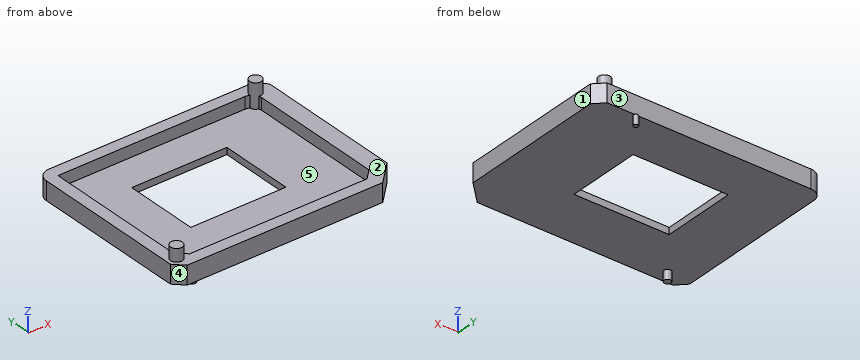
Autodesk Inventor part; units mm, degrees
ref_plane "YZ Plane" through (0, 0, 0) normal (1, 0, 0) x (0, 1, 0)
ref_plane "XZ Plane" through (0, 0, 0) normal (0, 1, 0) x (-1, 0, 0)
ref_plane "XY Plane" through (0, 0, 0) normal (0, 0, 1) x (1, 0, 0)
sketch "Sketch1" plane through (0, 0, 0) normal (0, 0, 1) x (1, 0, 0)
  line L0 (2, 0) -> (43.86, 0)
  line L1 (48.26, 4.4) -> (48.26, 36.1)
  line L2 (46.26, 38.1) -> (2.6, 38.1)
  line L3 (0, 35.5) -> (0, 2)
  arc A0 (2.6, 38.1) -> (0, 35.5) centre (2.6, 35.5) ccw
  line L4 (2.54, 35.56) -> (42.54, 35.56)
  line L5 (44.54, 33.56) -> (44.54, 4.56)
  line L6 (42.54, 2.56) -> (4.54, 2.56)
  line L7 (2.54, 4.56) -> (2.54, 35.56)
  line L8 (43.86, 0) -> (48.26, 4.4)
  line L9 (44.54, 4.56) -> (42.54, 2.56)
  line L10 (4.54, 2.56) -> (2.54, 4.56)
  circle A1 centre (44.72, 35.43) radius 1.28
  circle A2 centre (1.97, 2.85) radius 1.27
  line L11 (2.54, 35.56) -> (44.54, 2.56) construction
  line L12 (44.54, 35.56) -> (2.54, 2.56) construction
  arc A3 (44.54, 33.56) -> (42.54, 35.56) centre (42.54, 33.56) ccw
  line L13 (48.26, 36.1) -> (46.26, 38.1)
  line L14 (2, 0) -> (0, 2)
  point P0 (0, 0)
  point P1 (48.26, 38.1)
  point P2 (48.26, 0)
  point P3 (0, 38.1)
  point P4 (4.2502, 2.8498)
  point P5 (2.916, 4.184)
  point P6 (43.4429, 35.3446)
  point P7 (44.4412, 34.1807)
  dimension "d0" = 38.1
  dimension "d1" = 48.26
  dimension "d2" = 2.6
  dimension "d3" = 33
  dimension "d4" = 42
  dimension "d5" = 2.54
  dimension "d6" = 2.54
  dimension "d7" = 4.4
  dimension "d8" = 4.4
  dimension "d9" = 2
  dimension "d10" = 2
  dimension "d11" = 2
  dimension "d12" = 2
  dimension "d13" = 44.72
  dimension "d14" = 2.56
  dimension "d15" = 2.67
  dimension "d16" = 2.54
  dimension "d27" = 2
  dimension "d28" = 2
  dimension "d29" = 2
  dimension "d30" = 1.97
  dimension "d31" = 2.85
  dimension "d32" = 2
  dimension "d33" = 2
extrude "Extrusion1" add sketch "Sketch1" along normal blind 1.43 contours L14 L3 A0 L2 L13 L1 L8 L0 | L4 A3 A1 L5 L9 L6 L10 L7 | A3 A1 | A1 A3 | A2
extrude "Extrusion2" add sketch "Sketch1" along normal blind 3.95
extrude "Extrusion3" add sketch "Sketch1" along normal blind 4 contours A3 A1 | A1 A3 | A2
extrude "Extrusion4" add sketch "Sketch1" along normal blind 6.66 contours A3 A1 | A1 A3 | A2
sketch "Sketch2" plane through (0, 0, 1.43) normal (0, 0, 1) x (1, 0, 0)
  line L0 (12.36, 28.032) -> (32.72, 28.032)
  line L1 (32.72, 28.032) -> (32.72, 12.088)
  line L2 (32.72, 12.088) -> (12.36, 12.088)
  line L3 (12.36, 12.088) -> (12.36, 28.032)
  line L4 (2.54, 35.56) -> (42.54, 35.56)
  line L5 (2.54, 4.56) -> (2.54, 35.56)
  point P0 (0, 0)
  point P1 (22.54, 28.032)
  point P2 (22.54, 35.56)
  point P3 (2.54, 20.06)
  point P4 (12.36, 20.06)
  dimension "d34" = 25.86
  dimension "d35" = 20.36
extrude "Extrusion5" cut sketch "Sketch2" against normal blind 4
sketch "Sketch3" plane through (0, 0, 0) normal (0, 0, -1) x (-1, 0, 0)
  circle A0 centre (-39.96, 37.888) radius 0.4997
  circle A1 centre (-5.36, 2.788) radius 0.73
  line L0 (-2, 0) -> (-43.86, 0)
  line L1 (0, 35.5) -> (0, 2)
  line L2 (-46.26, 38.1) -> (-2.6, 38.1)
  line L3 (-12.36, 12.088) -> (-12.36, 28.032)
  point P0 (0, 0)
  dimension "d40" = 1.46
  dimension "d45" = 34.6
  dimension "d46" = 35.1
  dimension "d47" = 7
  dimension "d48" = 9.3
extrude "Extrusion6" add sketch "Sketch3" along normal blind 2
equation "\"d10\" = d9"
equation "\"d12\" = d11"
properties part number "tray"
Work out the finished part from the listing and answer in its coordinate system (mm). Face numbers are marked on the shaded views. A direction names the side the tool comes from. Give positions to 0.01 mm unless a question says otherwise; leave off trailing zeros. Write each loop counter-clockwise with the first axis right and the second up, starting at its lowest first coordinate (ties: lowest second). Pieces come first, ordered by that corner, then holes.
(1) The mould has two halves that part along X. Classify the marked faces 3, 4 and 5: pulls with the +X half, pulls with the -X half, needs draft (parallel to the pull), parting line crosses it, or undercut.
Final values:
face 3: needs draft
face 4: pulls with the -X half
face 5: undercut
(2) The part is cut by section D-D on x = 5.36. Write down the section's boundary in (y, z), plus the area to 3 significant figures.
Final values:
outline: (0, 0) - (2.06, 0) - (2.06, -2) - (3.52, -2) - (3.52, 0) - (38.1, 0) - (38.1, 3.95) - (35.56, 3.95) - (35.56, 1.43) - (2.56, 1.43) - (2.56, 3.95) - (0, 3.95) - close
area: 70.3 mm2
(3) The part is cut by section C-C on z = 4.75. Write down the section's boundary in (x, y).
Final values:
outline: circle Ø2.54 at (1.97, 2.85); circle Ø2.56 at (44.72, 35.43)
(4) The part is cut by section A-A on y = 16.5. Write down the section's boundary in (x, z).
Final values:
outline: (0, 0) - (12.36, 0) - (12.36, 1.43) - (2.54, 1.43) - (2.54, 3.95) - (0, 3.95) - close; (32.72, 0) - (48.26, 0) - (48.26, 3.95) - (44.54, 3.95) - (44.54, 1.43) - (32.72, 1.43) - close
(5) Flat-ended cylindrical pins translate along their axes: pin 1 Ø4 at (x, y) = (29.5, 20.5) entering from +Z; pin 2 Ø1.5 at (x, y) = (6.5, 10.5) entering from +Z; pin 3 Ø4 at (y, z) = (31.5, 2) entering from -X; pin 4 Ø19 at (x, y) = (25.5, 11) entering from +Z. Find the tip coordinate at first contact, or state that the pin passes through.
Final values:
pin 1: passes through
pin 2: stops at z = 1.43
pin 3: stops at x = 0
pin 4: stops at z = 3.95
(6) Which of the six approach directions +Z, -Z, +X, -X, +Y, -Y give full straight-line access (tool end or side, diameter ignored) to the marked faces 1 and 2?
Final values:
face 1: +Z, -Z, +X, +Y, -Y
face 2: +Z
(7) The part is cut by section B-B on x = 19. Write down the section's boundary in (y, z).
Final values:
outline: (0, 0) - (12.09, 0) - (12.09, 1.43) - (2.56, 1.43) - (2.56, 3.95) - (0, 3.95) - close; (28.03, 0) - (38.1, 0) - (38.1, 3.95) - (35.56, 3.95) - (35.56, 1.43) - (28.03, 1.43) - close
(8) Straight lines are drawn through the part: line 1 (X direction, y = 14, z = 1.75); line 2 (Y direction, x = 31, z = 3.75); line 3 (Y direction, x = 11, z = 0.75). For each, find the intervals that lie inside material, in ascending order.
Final values:
line 1: x = 0 to 2.54, 44.54 to 48.26
line 2: y = 0 to 2.56, 35.56 to 38.1
line 3: y = 0 to 38.1
